The drawing under review shows one solid part. Ordinate dimensions are in mm from its lowest x, y, z. A direction names the side the tool comes from. Give positions to 0.01 mm unless a question says otherwise; leave off trailing zeros. Order: outer loops, then holes, each group sorted by start corner. A loop starts at its lowest first (then second) coordinate and runs counter-clockwise, first axis right, second up. Notation, with made-up numbers: (-7, -20.75) -> (50, -20.75) arc R17 cw to (50, -11.75) -> close; hole circle Ø10 at (-36, 9). An arc over 180 degrees is marked (long way). Use a Markdown table: item, result. Add a question column.
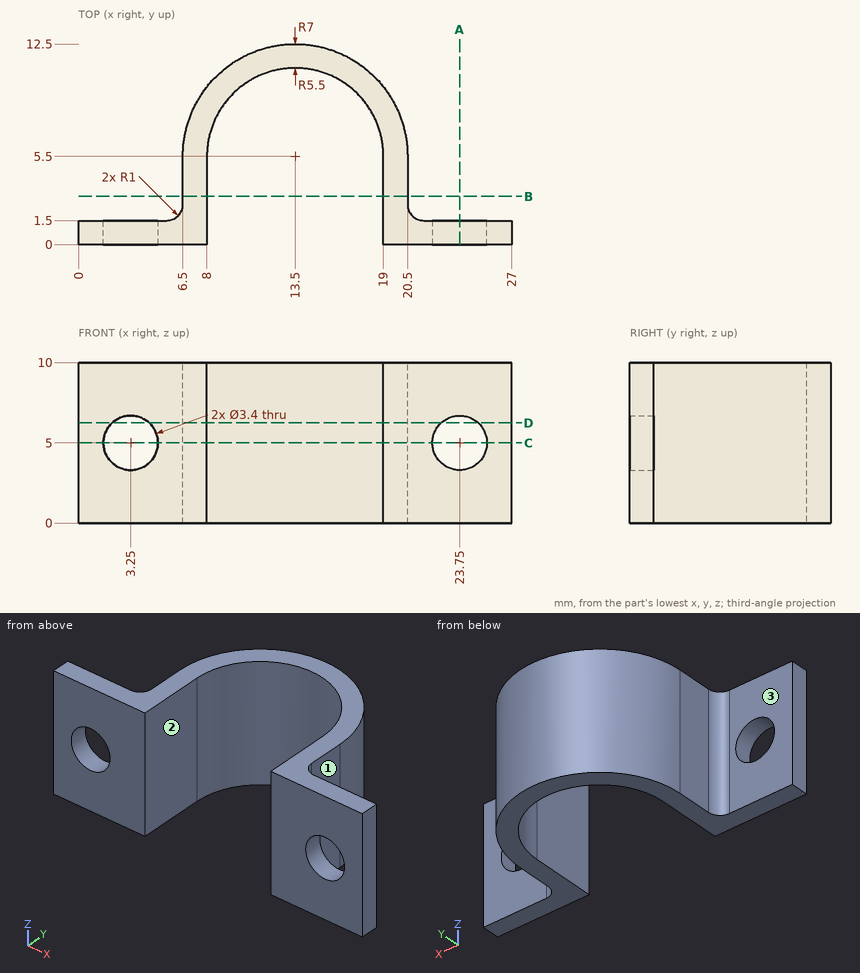
1) Insertion check: pin 1 (1 mm diameter, centred on y = 11, z = 1.5, fed in from +X); pin 2 (4 mm diameter, centred on y = 6.5, z = 4, fed in from +X); pin 3 (4.5 mm diameter, centred on x = 24.5, z = 4, fed in from +Y); pin 4 (2.5 mm diameter, centred on x = 3.25, z = 5, fed in from +Y). Each pin has a flat end and moves straight along its axis. Give the tip position at first contact, or say it passes through.
2) For L1, parallel to X at y = 3, z = 1.5; L2, parallel to Z at x = 23.75, y = 0.95; L3, parallel to Y at x = 21.5, z = 1.5, list the stretches that pass through material, from the lowest coordinate up. Write a range as [from, to].
3) Add section D-D (z = 6.25). Give the boundary of the cut face in (x, y).
4) Add section B-B (y = 3). Give the boundary of the cut face in (x, z).
5) Add section A-A (x = 23.75). Give the boundary of the cut face in (y, z), then the cut area to 3 significant figures.
6) Add section C-C (z = 5). Give the boundary of the cut face in (x, y).
7) Machinability: for the marked faces 1, 2 and 3, which of the approach directions +Z, -Z, +X, -X, +Y, -Y give a long, thin tool a straight path to every point of the face, cutting with its end or side? Answer none if there is none.
Worked answers:
| question | item | result |
|---|---|---|
| 1 | pin 1 | x = 18.4 |
| 1 | pin 2 | x = 20.5 |
| 1 | pin 3 | y = 1.5 |
| 1 | pin 4 | through |
| 2 | L1 | [6.5, 8], [19, 20.5] |
| 2 | L2 | [0, 3.3], [6.7, 10] |
| 2 | L3 | [0, 1.5] |
| 3 | outline | (0, 0) -> (2.1, 0) -> (2.1, 1.5) -> (0, 1.5) -> close; (4.4, 0) -> (8, 0) -> (8, 5.5) arc R5.5 cw to (19, 5.5) -> (19, 0) -> (22.6, 0) -> (22.6, 1.5) -> (21.5, 1.5) arc R1 cw to (20.5, 2.5) -> (20.5, 5.5) arc R7 ccw to (6.5, 5.5) -> (6.5, 2.5) arc R1 cw to (5.5, 1.5) -> (4.4, 1.5) -> close; (24.9, 0) -> (27, 0) -> (27, 1.5) -> (24.9, 1.5) -> close |
| 4 | outline | (6.5, 0) -> (8, 0) -> (8, 10) -> (6.5, 10) -> close; (19, 0) -> (20.5, 0) -> (20.5, 10) -> (19, 10) -> close |
| 5 | outline | (0, 0) -> (1.5, 0) -> (1.5, 3.3) -> (0, 3.3) -> close; (0, 6.7) -> (1.5, 6.7) -> (1.5, 10) -> (0, 10) -> close |
| 5 | area | 9.90 mm^2 |
| 6 | outline | (0, 0) -> (1.55, 0) -> (1.55, 1.5) -> (0, 1.5) -> close; (4.95, 0) -> (8, 0) -> (8, 5.5) arc R5.5 cw to (19, 5.5) -> (19, 0) -> (22.05, 0) -> (22.05, 1.5) -> (21.5, 1.5) arc R1 cw to (20.5, 2.5) -> (20.5, 5.5) arc R7 ccw to (6.5, 5.5) -> (6.5, 2.5) arc R1 cw to (5.5, 1.5) -> (4.95, 1.5) -> close; (25.45, 0) -> (27, 0) -> (27, 1.5) -> (25.45, 1.5) -> close |
| 7 | face 1 | +Z, -Z, +X, +Y |
| 7 | face 2 | +Z, -Z, -Y |
| 7 | face 3 | +Z, -Z, -X, +Y |
